CAD build for the part. Positions are in the model's coordinates, mm. Face numbers are marked on the shaded views. A direction names the side the tool comes from. Coordinates: 2 decimals unless noted, no trailing zeros. Loops run counter-clockwise (first coordinate to the right, second up) from the corner with the lowest first, then second, coordinate; pieces in that order, holes last. Notation, with made-up numbers: (-30, 74) -> (-14, 74) arc R29 ccw to (-14, 110) -> close; hole circle Ø3 at (13, 31.5). An arc over 180 degrees is marked (long way). Answer as a JSON object with one key per item and string values. Group by question number.
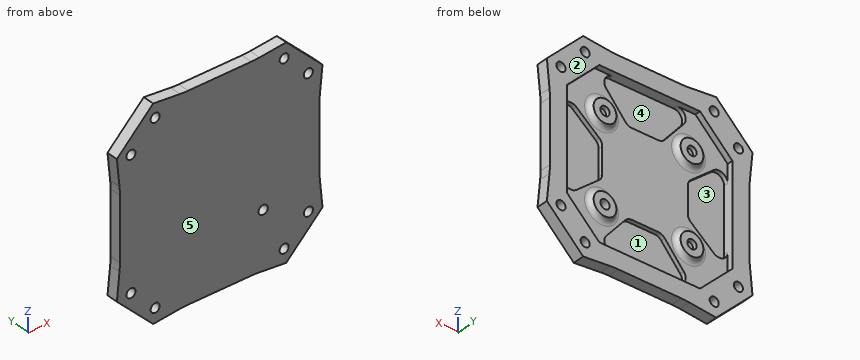
from build123d import *

# Parameters (mm, degrees)
SKETCH1_R           = 1.6
BOSS_EXTRUDE2_DEPTH = 4
CUT_EXTRUDE1_DEPTH  = 2
CUT_EXTRUDE2_DEPTH  = 1.5
SKETCH4_R           = 1.625
CUT_EXTRUDE3_DEPTH  = 52.039200621
BOSS_EXTRUDE3_START = 1.5
SKETCH5_R           = 4
SKETCH5_R_2         = 1.625
BOSS_EXTRUDE3_DEPTH = 1.5
CIRPATTERN1_COUNT   = 4
FILLET1_R           = 2
FILLET2_R           = 30


with BuildPart() as part:
    # Sketch1 → Boss-Extrude2 (new body)
    with BuildSketch(Plane(origin=(0, 0, 0), x_dir=(1, 0, 0), z_dir=(0, 1, 0))):
        Polygon((-12.5, 35), (12.5, 35), (23.334523779, 36.062445841), (36.062445841, 23.334523779), (35, 12.5), (35, -12.5), (36.062445841, -23.334523779), (23.334523779, -36.062445841), (12.5, -35), (-12.5, -35), (-23.334523779, -36.062445841), (-36.062445841, -23.334523779), (-35, -12.5), (-35, 12.5), (-36.062445841, 23.334523779), (-23.334523779, 36.062445841), align=None)
        with Locations(Location((22.627416998, 31.112698372, 0), (0, 0, 270))):
            Circle(SKETCH1_R, mode=Mode.SUBTRACT)
        with Locations(Location((31.112698372, 22.627416998, 0), (0, 0, 270))):
            Circle(SKETCH1_R, mode=Mode.SUBTRACT)
        with Locations(Location((22.627416998, -31.112698372, 0), (0, 0, 270))):
            Circle(SKETCH1_R, mode=Mode.SUBTRACT)
        with Locations(Location((31.112698372, -22.627416998, 0), (0, 0, 270))):
            Circle(SKETCH1_R, mode=Mode.SUBTRACT)
        with Locations(Location((-31.112698372, -22.627416998, 0), (0, 0, 270))):
            Circle(SKETCH1_R, mode=Mode.SUBTRACT)
        with Locations(Location((-22.627416998, -31.112698372, 0), (0, 0, 270))):
            Circle(SKETCH1_R, mode=Mode.SUBTRACT)
        with Locations(Location((-22.627416998, 31.112698372, 0), (0, 0, 270))):
            Circle(SKETCH1_R, mode=Mode.SUBTRACT)
        with Locations(Location((-31.112698372, 22.627416998, 0), (0, 0, 270))):
            Circle(SKETCH1_R, mode=Mode.SUBTRACT)
    extrude(amount=BOSS_EXTRUDE2_DEPTH)

    # Sketch2 → Cut-Extrude1 (cut)
    with BuildSketch(Plane(origin=(0, 4, 0), x_dir=(1, 0, 0), z_dir=(0, 1, 0))):
        Polygon((-17.669047558, 29), (17.669047558, 29), (29, 17.669047558), (29, -17.669047558), (17.669047558, -29), (-17.669047558, -29), (-29, -17.669047558), (-29, 17.669047558), align=None)
    extrude(amount=-CUT_EXTRUDE1_DEPTH, mode=Mode.SUBTRACT)

    # Sketch3 → Cut-Extrude2 (cut)
    with BuildSketch(Plane(origin=(0, 2, 0), x_dir=(1, 0, 0), z_dir=(0, 1, 0))):
        with BuildLine():
            Line((-24.079215521, 13.567556979), (-16.079215521, 6.899529803))
            ThreePointArc((-16.079215521, 6.899529803), (-15.283167889, 5.867388581), (-15, 4.595058717))
            Line((-15, 4.595058717), (-15, -4.595058717))
            ThreePointArc((-15, -4.595058717), (-15.283167889, -5.867388581), (-16.079215521, -6.899529803))
            Line((-16.079215521, -6.899529803), (-24.079215521, -13.567556979))
            ThreePointArc((-24.079215521, -13.567556979), (-27.272329864, -13.979918004), (-29, -11.263085893))
            Line((-29, -11.263085893), (-29, 11.263085893))
            ThreePointArc((-29, 11.263085893), (-27.272329864, 13.979918004), (-24.079215521, 13.567556979))
        make_face()
        with BuildLine():
            Line((13.567556979, 24.079215521), (6.899529803, 16.079215521))
            ThreePointArc((6.899529803, 16.079215521), (5.867388581, 15.283167889), (4.595058717, 15))
            Line((4.595058717, 15), (-4.595058717, 15))
            ThreePointArc((-4.595058717, 15), (-5.867388581, 15.283167889), (-6.899529803, 16.079215521))
            Line((-6.899529803, 16.079215521), (-13.567556979, 24.079215521))
            ThreePointArc((-13.567556979, 24.079215521), (-13.979918004, 27.272329864), (-11.263085893, 29))
            Line((-11.263085893, 29), (11.263085893, 29))
            ThreePointArc((11.263085893, 29), (13.979918004, 27.272329864), (13.567556979, 24.079215521))
        make_face()
        with BuildLine():
            Line((24.079215521, -13.567556979), (16.079215521, -6.899529803))
            ThreePointArc((16.079215521, -6.899529803), (15.283167889, -5.867388581), (15, -4.595058717))
            Line((15, -4.595058717), (15, 4.595058717))
            ThreePointArc((15, 4.595058717), (15.283167889, 5.867388581), (16.079215521, 6.899529803))
            Line((16.079215521, 6.899529803), (24.079215521, 13.567556979))
            ThreePointArc((24.079215521, 13.567556979), (27.272329864, 13.979918004), (29, 11.263085893))
            Line((29, 11.263085893), (29, -11.263085893))
            ThreePointArc((29, -11.263085893), (27.272329864, -13.979918004), (24.079215521, -13.567556979))
        make_face()
        with BuildLine():
            Line((-13.567556979, -24.079215521), (-6.899529803, -16.079215521))
            ThreePointArc((-6.899529803, -16.079215521), (-5.867388581, -15.283167889), (-4.595058717, -15))
            Line((-4.595058717, -15), (4.595058717, -15))
            ThreePointArc((4.595058717, -15), (5.867388581, -15.283167889), (6.899529803, -16.079215521))
            Line((6.899529803, -16.079215521), (13.567556979, -24.079215521))
            ThreePointArc((13.567556979, -24.079215521), (13.979918004, -27.272329864), (11.263085893, -29))
            Line((11.263085893, -29), (-11.263085893, -29))
            ThreePointArc((-11.263085893, -29), (-13.979918004, -27.272329864), (-13.567556979, -24.079215521))
        make_face()
    extrude(amount=-CUT_EXTRUDE2_DEPTH, mode=Mode.SUBTRACT)

    # Sketch4 → Cut-Extrude3 (cut, through all)
    with BuildSketch(Plane(origin=(0, 2, 0), x_dir=(1, 0, 0), z_dir=(0, 1, 0))):
        with Locations(Location((15.25, 15.25, 0), (0, 0, 270))):
            Circle(SKETCH4_R)
    extrude(amount=-CUT_EXTRUDE3_DEPTH, mode=Mode.SUBTRACT)

    # Sketch5 → Boss-Extrude3 (add)
    with BuildSketch(Plane(origin=(0, 2, 0), x_dir=(1, 0, 0), z_dir=(0, 1, 0)).offset(BOSS_EXTRUDE3_START)):
        with Locations(Location((15.25, 15.25, 0), (0, 0, 90))):
            Circle(SKETCH5_R)
        with Locations(Location((15.25, 15.25, 0), (0, 0, 270))):
            Circle(SKETCH5_R_2, mode=Mode.SUBTRACT)
    boss_extrude3 = extrude(amount=-BOSS_EXTRUDE3_DEPTH)

    # CirPattern1: Boss-Extrude3 ×4 about axis
    cirpattern1_axis = Axis((0, 0, 0), (0, 1, 0))
    for i in range(1, CIRPATTERN1_COUNT):
        add(boss_extrude3.rotate(cirpattern1_axis, i * 360 / CIRPATTERN1_COUNT))

    # Fillet1
    # the kernel refuses this fillet: 2 mm, written as the material it adds along each edge
    with BuildSketch(Plane(origin=(15.25, 2, -15.25), x_dir=(0, 0, -1), z_dir=(1, 0, 0))) as fillet1_piece_1:
        with BuildLine():
            CenterArc((5.936491673, 2), FILLET1_R, 194.477512186, 75.522487814)
            Line((4, 1.5), (3.961270167, 1.49))
            ThreePointArc((3.961270167, 1.49), (3.96, 0.75), (3.96, 0))
            Line((3.96, 0), (4, -0.04))
            Line((4, -0.04), (5.936491673, -0.04))
            Line((5.936491673, -0.04), (5.936491673, 0))
        make_face()
    revolve(axis=Axis((15.25, 2, -15.25), (0, 1, 0)))
    with BuildSketch(Plane(origin=(15.25, 2, 15.25), x_dir=(1, 0, 0), z_dir=(0, 0, 1))) as fillet1_piece_2:
        with BuildLine():
            CenterArc((5.936491673, 2), FILLET1_R, 194.477512186, 75.522487814)
            Line((4, 1.5), (3.961270167, 1.49))
            ThreePointArc((3.961270167, 1.49), (3.96, 0.75), (3.96, 0))
            Line((3.96, 0), (4, -0.04))
            Line((4, -0.04), (5.936491673, -0.04))
            Line((5.936491673, -0.04), (5.936491673, 0))
        make_face()
    revolve(axis=Axis((15.25, 2, 15.25), (0, 1, 0)))
    with BuildSketch(Plane(origin=(-15.25, 2, 15.25), x_dir=(0, 0, 1), z_dir=(-1, 0, 0))) as fillet1_piece_3:
        with BuildLine():
            CenterArc((5.936491673, 2), FILLET1_R, 194.477512186, 75.522487814)
            Line((4, 1.5), (3.961270167, 1.49))
            ThreePointArc((3.961270167, 1.49), (3.96, 0.75), (3.96, 0))
            Line((3.96, 0), (4, -0.04))
            Line((4, -0.04), (5.936491673, -0.04))
            Line((5.936491673, -0.04), (5.936491673, 0))
        make_face()
    revolve(axis=Axis((-15.25, 2, 15.25), (0, 1, 0)))
    with BuildSketch(Plane(origin=(-15.25, 2, -15.25), x_dir=(-1, 0, 0), z_dir=(0, 0, -1))) as fillet1_piece_4:
        with BuildLine():
            CenterArc((5.936491673, 2), FILLET1_R, 194.477512186, 75.522487814)
            Line((4, 1.5), (3.961270167, 1.49))
            ThreePointArc((3.961270167, 1.49), (3.96, 0.75), (3.96, 0))
            Line((3.96, 0), (4, -0.04))
            Line((4, -0.04), (5.936491673, -0.04))
            Line((5.936491673, -0.04), (5.936491673, 0))
        make_face()
    revolve(axis=Axis((-15.25, 2, -15.25), (0, 1, 0)))

    # Fillet2
    # the kernel refuses this fillet: 30 mm, written as the material it adds along each edge
    with BuildSketch(Plane(origin=(-12.5, 0, -35), x_dir=(1, 0, 0), z_dir=(0, 1, 0)), Plane(origin=(-12.5, 0, 35), x_dir=(-0.995226405289247, 0, 0.09759304388655687), z_dir=(0, 1, 0)), Plane(origin=(-35, 0, 12.5), x_dir=(0, 0, -1), z_dir=(0, 1, 0)), Plane(origin=(-35, 0, -12.5), x_dir=(-0.09759304388656588, 0, -0.9952264052892461), z_dir=(0, 1, 0))) as fillet2_piece_1:
        with BuildLine():
            CenterArc((FILLET2_R * 0.0489132680017, FILLET2_R), FILLET2_R, 264.399415997, 5.600584003)
            Line((-FILLET2_R * 0.0486797758843, FILLET2_R * 0.0047735947107), (0, 0))
            Line((0, 0), (FILLET2_R * 0.0489132680017, 0))
        make_face()
    extrude(amount=4)
    with BuildSketch(Plane(origin=(12.5, 0, -35), x_dir=(-1, 0, 0), z_dir=(0, 1, 0)), Plane(origin=(35, 0, -12.5), x_dir=(0.09759304388597295, 0, -0.9952264052893043), z_dir=(0, 1, 0)), Plane(origin=(35, 0, 12.5), x_dir=(0, 0, -1), z_dir=(0, 1, 0)), Plane(origin=(12.5, 0, 35), x_dir=(0.9952264052893042, 0, 0.09759304388597305), z_dir=(0, 1, 0))) as fillet2_piece_2:
        with BuildLine():
            CenterArc((FILLET2_R * 0.048913268002, -FILLET2_R), FILLET2_R, 90, 5.600584003)
            Line((-FILLET2_R * 0.0486797758846, -FILLET2_R * 0.00477359471075), (0, 0))
            Line((0, 0), (FILLET2_R * 0.048913268002, 0))
        make_face()
    extrude(amount=4)


solid = part.part
Item 1: 3-axis set-ups, long thin cutter, end or side, ignore diameter. For the marked faces 1 and 2: which of +Z, -Z, +X, -X, +Y, -Y reach the whole face in a straight line?
Item 2: Band-saw the part on B-B, the plane y = 2.6. Count the separate pieces of the cut face and the enclosed holes in it, and give its area (3 significant figures).
Item 3: Band-saw the part on A-A, the plane x = -3.5. List the corners of the cut face in (y, z).
Item 4: Drill centre lines: L1, parallel to X at y = 1.3, z = 2.5; L2, parallel to X at y = 3.5, z = 11; L3, parallel to X at y = 1.05, z = -22.5. Where is each one in solid material? Low to high.
Item 5: Flat gauge pins, fed straight in: P1, Ø2, axis at x = -25, y = 1, coming from the -Z side; P2, Ø2, axis at x = 7, y = 2, coming from the -Z side; P3, Ø7, axis at x = -25, z = -0.5, coming from the +Y side. Where does each tip first touch, or does it go through?
Item 6: Pull direction Z, two halves, no side cores. Call the marked faces 3, 4 and 5: +Z half, -Z half, draft (parallel to the pull), parting line (faces both ways), or undercut.
Reply:
{
 "1": {"face 1": "+Y", "face 2": "+Z, -Z, +X, -X, +Y"},
 "2": {"separate pieces": "5", "enclosed holes": "13", "area": "1,780 mm²"},
 "3": {"outline": "(0, -35) -> (4, -35) -> (4, -29) -> (0.5, -29) -> (0.5, -15) -> (2, -15) -> (2, 15) -> (0.5, 15) -> (0.5, 29) -> (4, 29) -> (4, 35) -> (0, 35) -> close"},
 "4": {"L1": "-35 to -29, -15 to 15, 29 to 35", "L2": "-35 to -29, 29 to 35", "L3": "-35.98 to -32.71, -29.52 to -12.25, 12.25 to 29.52, 32.71 to 35.98"},
 "5": {"P1": "z = -35.4", "P2": "z = -35", "P3": "y = 0.5"},
 "6": {"face 3": "undercut", "face 4": "undercut", "face 5": "draft"}
}
